```python
from build123d import *

# Parameters (mm, degrees)
F0_R     = 6
F1_DEPTH = 15
F3_DEPTH = 12
F5_DEPTH = 18.5


with BuildPart() as f1:
    # F0 (on Top) → F1 (new body, symmetric)
    with BuildSketch(Plane.XY):
        Circle(F0_R)
    extrude(amount=F1_DEPTH, both=True)

    # F2 (on face) → F3 (cut)
    with BuildSketch(Plane(origin=(0, 0, -15), x_dir=(1, 0, 0), z_dir=(0, 0, -1))):
        with BuildLine():
            Line((-1.9798989873, -2.45), (1.9798989873, -2.45))
            ThreePointArc((1.9798989873, -2.45), (0, 3.15), (-1.9798989873, -2.45))
        make_face()
    extrude(amount=-F3_DEPTH, mode=Mode.SUBTRACT)

    # F4 (on face) → F5 (cut)
    with BuildSketch(Plane.XY.offset(15)):
        Polygon((-1.9485571585, -3.375), (1.9485571585, -3.375), (3.897114317, 0), (1.9485571585, 3.375), (-1.9485571585, 3.375), (-3.897114317, 0), align=None)
    extrude(amount=-F5_DEPTH, mode=Mode.SUBTRACT)


solid = f1.part
```
Input: part model. Units: mm. Frame: model coordinates. A direction names the side the tool comes from. Coordinates: 2 decimals unless noted, no trailing zeros. Loops run counter-clockwise (first coordinate to the right, second up) from the corner with the lowest first, then second, coordinate; pieces in that order, holes last. Notation, with made-up numbers: M 86.25,-4.75 L 128.25,-4.75 A32 ccw 128.25,32.25 Z; hole C 45,53 d1. An arc over 180 degrees is marked long. One line per item, written item: value.
(1) Section D-D (y = 4.5). Output: boundary loops of the cut face in (x, z).
Filled in:
outline: M -3.97,-15 L 3.97,-15 L 3.97,15 L -3.97,15 Z
(2) Pull-direction query (X, two-part tool) for faces 4 (the flat face through (-2.91, 1.71, 5.88)), 5 (the flat face through (0, 3, -15)), 6 (the cylindrical face through (0.11, -3.15, -9.33)), 7 (the cylindrical face through (-6, 0, 0)); classes: +X half, -X half, draft (parallel to the pull), parting line (faces both ways), or undercut.
Filled in:
face 4: undercut
face 5: draft
face 6: undercut
face 7: parting line
(3) Section C-C (x = -1.5). Output: boundary loops of the cut face in (y, z) (3 decimals), and give its area (3 significant figures).
Filled in:
outline: M -5.809,-15 L -2.77,-15 L -2.77,-3.5 L -3.375,-3.5 L -3.375,15 L -5.809,15 Z; M 2.45,-15 L 5.809,-15 L 5.809,15 L 3.375,15 L 3.375,-3.5 L 2.45,-3.5 Z
area: 164 mm^2
(4) Reachability of faces 1 (the flat face through (3, -3, 15)), 2 (the flat face through (0, 2.45, -9)), 3 (the flat face through (0, 3, -3.5)) from +Z, -Z, +X, -X, +Y, -Y: full face, straight path, thin tool, end or side. Return the list, or none.
Filled in:
face 1: +Z, +X, -X, +Y, -Y
face 2: +Z, -Z
face 3: +Z
(5) Line query: line 1 along Y through (x, z) = (0, -6.25); line 2 along X through (y, z) = (-2.5, 11); line 3 along X through (y, z) = (-0.5, -9.75). Output: solid intervals per line, ascending. Write a range as from..to.
Filled in:
line 1: -6..-3.15, 2.45..6
line 2: -5.45..-2.45, 2.45..5.45
line 3: -5.98..-3.11, 3.11..5.98
(6) Pin query (flat end, axial travel): pin 1 (6 mm diameter, centred on y = -3.5, z = -1.5, fed in from +X); pin 2 (5 mm diameter, centred on x = 3.5, z = -12, fed in from +Y); pin 3 (4 mm diameter, centred on y = -3.5, z = -7.5, fed in from +X). Return the tip coordinate at first contact, or that it passes through.
Filled in:
pin 1: x = 5.98
pin 2: y = 5.92
pin 3: x = 5.81
(7) Section B-B (x = 0). Output: boundary loops of the cut face in (y, z) (3 decimals), and give its area (3 significant figures).
Filled in:
outline: M -6,-15 L -3.15,-15 L -3.15,-3.5 L -3.375,-3.5 L -3.375,15 L -6,15 Z; M 2.45,-15 L 6,-15 L 6,15 L 3.375,15 L 3.375,-3.5 L 2.45,-3.5 Z
area: 171 mm^2
(8) Section A-A (z = 8.25). Output: boundary loops of the cut face in (x, y) (3 decimals).
Filled in:
outline: C 0,0 d12; hole M -3.897,0 L -1.949,-3.375 L 1.949,-3.375 L 3.897,0 L 1.949,3.375 L -1.949,3.375 Z
